```python
from build123d import *

# Parameters (mm, degrees)
EXTRUDE_1_DEPTH             = 90
SKETCH_2_W                  = 90
SKETCH_2_H                  = 17.75
EXTRUDE_2_DEPTH             = 8.2
SKETCH_3_W                  = 90
SKETCH_3_H                  = 50.95
EXTRUDE_3_DEPTH             = 8.2
SKETCH_4_W                  = 3.95
SKETCH_4_H                  = 29.5
CUT_EXTRUDE_1_DEPTH         = 91
SKETCH_5_W                  = 3.95
SKETCH_5_H                  = 6.2
CUT_EXTRUDE_2_DEPTH         = 91
SKETCH_6_W                  = 2.25
SKETCH_6_H                  = 3.95
CUT_EXTRUDE_3_DEPTH         = 91
SKETCH_7_W                  = 4.5
SKETCH_7_H                  = 3.95
CUT_EXTRUDE_4_DEPTH         = 91
SKETCH_8_W                  = 2.25
SKETCH_8_H                  = 3.95
CUT_EXTRUDE_5_DEPTH         = 91
SKETCH_9_W                  = 3.95
SKETCH_9_H                  = 2.25
CUT_EXTRUDE_6_DEPTH         = 91
SKETCH_10_W                 = 19.6
SKETCH_10_H                 = 44.6
CUT_EXTRUDE_7_DEPTH         = 86.2
HOLE_WIZARD_2_5_2_5_1_D     = 2.5
HOLE_WIZARD_2_5_2_5_1_DEPTH = 90
HOLE_WIZARD_4_5_4_5_1_D     = 4.5
HOLE_WIZARD_4_5_4_5_1_DEPTH = 90
FILLET_1_R                  = 2
FILLET_2_R                  = 2
SKETCH_17_R                 = 1.25
EXTRUDE_4_DEPTH             = 90


with BuildPart() as part:
    # Эскиз1 → Бобышка-Вытянуть1 (new body)
    with BuildSketch(Plane(origin=(90, 0, 0), x_dir=(0, 0, -1), z_dir=(1, 0, 0))):
        with BuildLine():
            Line((6.75, -24.093761792), (6.75, 19.25))
            Line((6.75, 19.25), (-11.593761792, 19.25))
            ThreePointArc((-11.593761792, 19.25), (-15.325, 18), (-11.593761792, 16.75))
            Line((-11.593761792, 16.75), (-11, 16.75))
            Line((-11, 16.75), (-11, -16.75))
            Line((-11, -16.75), (-11.593761792, -16.75))
            ThreePointArc((-11.593761792, -16.75), (-15.325, -18), (-11.593761792, -19.25))
            Line((-11.593761792, -19.25), (-11, -19.25))
            Line((-11, -19.25), (-11, -23.5))
            Line((-11, -23.5), (-6.75, -23.5))
            Line((-6.75, -23.5), (-6.75, -24.093761792))
            ThreePointArc((-6.75, -24.093761792), (-5.5, -27.825), (-4.25, -24.093761792))
            Line((-4.25, -24.093761792), (-4.25, -23.5))
            Line((-4.25, -23.5), (4.25, -23.5))
            Line((4.25, -23.5), (4.25, -24.093761792))
            ThreePointArc((4.25, -24.093761792), (5.5, -27.825), (6.75, -24.093761792))
        make_face()
    extrude(amount=-EXTRUDE_1_DEPTH)

    # Эскиз2 → Бобышка-Вытянуть2 (add)
    with BuildSketch(Plane(origin=(0, 19.25, 0), x_dir=(-1, 0, 0), z_dir=(0, 1, 0))):
        with Locations((-45, 2.125)):
            Rectangle(SKETCH_2_W, SKETCH_2_H)
    extrude(amount=EXTRUDE_2_DEPTH)

    # Эскиз3 → Бобышка-Вытянуть3 (add)
    with BuildSketch(Plane(origin=(0, 0, -6.75), x_dir=(-1, 0, 0), z_dir=(0, 0, -1))):
        with Locations((-45, 1.975)):
            Rectangle(SKETCH_3_W, SKETCH_3_H)
    extrude(amount=EXTRUDE_3_DEPTH)

    # Эскиз4 → Вырез-Вытянуть1 (cut, through all)
    with BuildSketch(Plane.ZY):
        with Locations((-12.975, 0)):
            Rectangle(SKETCH_4_W, SKETCH_4_H)
    extrude(amount=-CUT_EXTRUDE_1_DEPTH, mode=Mode.SUBTRACT)

    # Эскиз5 → Вырез-Вытянуть2 (cut, through all)
    with BuildSketch(Plane.ZY):
        with Locations((-12.975, 24.35)):
            Rectangle(SKETCH_5_W, SKETCH_5_H)
    extrude(amount=-CUT_EXTRUDE_2_DEPTH, mode=Mode.SUBTRACT)

    # Эскиз6 → Вырез-Вытянуть3 (cut, through all)
    with BuildSketch(Plane.ZY):
        with Locations((-9.875, 25.475)):
            Rectangle(SKETCH_6_W, SKETCH_6_H)
    extrude(amount=-CUT_EXTRUDE_3_DEPTH, mode=Mode.SUBTRACT)

    # Эскиз7 → Вырез-Вытянуть4 (cut, through all)
    with BuildSketch(Plane.ZY):
        with Locations((0, 25.475)):
            Rectangle(SKETCH_7_W, SKETCH_7_H)
    extrude(amount=-CUT_EXTRUDE_4_DEPTH, mode=Mode.SUBTRACT)

    # Эскиз8 → Вырез-Вытянуть5 (cut, through all)
    with BuildSketch(Plane.ZY):
        with Locations((9.875, 25.475)):
            Rectangle(SKETCH_8_W, SKETCH_8_H)
    extrude(amount=-CUT_EXTRUDE_5_DEPTH, mode=Mode.SUBTRACT)

    # Эскиз9 → Вырез-Вытянуть6 (cut, through all)
    with BuildSketch(Plane.ZY):
        with Locations((-12.975, -22.375)):
            Rectangle(SKETCH_9_W, SKETCH_9_H)
    extrude(amount=-CUT_EXTRUDE_6_DEPTH, mode=Mode.SUBTRACT)

    # Эскиз10 → Вырез-Вытянуть7 (cut)
    with BuildSketch(Plane(origin=(90, 0, 0), x_dir=(0, 0, -1), z_dir=(1, 0, 0))):
        Rectangle(SKETCH_10_W, SKETCH_10_H)
    extrude(amount=-CUT_EXTRUDE_7_DEPTH, mode=Mode.SUBTRACT)

    # Диаметр отверстия Ø2.5 (2.5)1
    with Locations(Plane(origin=(90, 0, 0), x_dir=(0, 0, -1), z_dir=(1, 0, 0))):
        with Locations((5.5, -25.75), (-13.25, -18), (-5.5, -25.75), (-13.25, 18)):
            Hole(HOLE_WIZARD_2_5_2_5_1_D / 2, depth=HOLE_WIZARD_2_5_2_5_1_DEPTH)

    # Диаметр отверстия Ø4.5 (4.5)1
    with Locations(Plane.ZY):
        with Locations((-13.25, -18), (-13.25, 18), (-5.5, 25.75), (5.5, 25.75)):
            Hole(HOLE_WIZARD_4_5_4_5_1_D / 2, depth=HOLE_WIZARD_4_5_4_5_1_DEPTH)

    # Скругление1
    fillet_1_edges = [part.edges().sort_by_distance(p)[0] for p in [
        (45, 23.5, 8.75),
    ]]
    fillet(fillet_1_edges, radius=FILLET_1_R)

    # Скругление2
    fillet_2_edges = [part.edges().sort_by_distance(p)[0] for p in [
        (45, 23.5, -8.75),
        (45, 23.5, 2.25),
        (45, 23.5, -2.25),
        (45, -21.25, -11),
        (45, 14.75, -11),
        (45, -14.75, -11),
        (45, 21.25, -11),
    ]]
    fillet(fillet_2_edges, radius=FILLET_2_R)

    # Эскиз17 → Бобышка-Вытянуть4 (add)
    with BuildSketch(Plane(origin=(90, 0, 0), x_dir=(0, 0, -1), z_dir=(1, 0, 0))):
        with Locations((5.5, -25.75)):
            Circle(SKETCH_17_R)
        with Locations((-5.5, -25.75)):
            Circle(SKETCH_17_R)
        with Locations((-13.25, -18)):
            Circle(SKETCH_17_R)
        with Locations((-13.25, 18)):
            Circle(SKETCH_17_R)
    extrude(amount=-EXTRUDE_4_DEPTH)


solid = part.part
```
Part model, mm, in its own coordinate system. A direction names the side the tool comes from. Round coordinates to 2 decimals unless told otherwise and drop trailing zeros. Order: outer loops, then holes, each group sorted by start corner. A loop starts at its lowest first (then second) coordinate and runs counter-clockwise, first axis right, second up. Notation, with made-up numbers: M 88.5,56 L 130.5,56 A12 cw 130.5,64 Z; hole C 0.25,52.5 d11. An arc over 180 degrees is marked long. Answer in a Markdown table with one row per item. Add a question column.
Q1. Cut at C-C on y = -6. Give the cut face in (x, z).
Q2. Cut at B-B on z = 13.25. Give the cut face in (x, y) (3 decimals).
Q3. 3-axis set-ups, long thin cutter, end or side, ignore diameter. For faces 1 (the face through (46, 21, 11)), 2 (the face through (45.63, -14.15, -11.57)), 3 (the face through (46, -23.5, 0)): which of +Z, -Z, +X, -X, +Y, -Y reach the whole face in a straight line?
Q4. Mould opens along Z. For faces 4 (the face through (48, 22.3, 0)), 5 (the face through (44, 26, -8.75)), 6 (the face through (44, 26, 8.75)), 7 (the face through (0, -1, 0)) say: +Z half, -Z half, draft (parallel to the pull), parting line (faces both ways), or undercut.
Q5. Cut at A-A on y = -25.75. Give the cut face in (x, z) (3 decimals), and give its area (3 significant figures).
Q6. Wall check: L1, parallel to Y at x = 44, z = -13.25; L2, parallel to Z at x = 29, y = 25.75; L3, parallel to Y at x = 50, z = -13. Give the ranges that are in metal, low to high. Write a range as from..to.
Q7. Cut at D-D on z = -5.5. Give the cut face in (x, y) (3 decimals).
Q8. Pin check, flat tips, straight feed: pin 1 (1.6 mm diameter, centred on x = 64.5, z = -14, fed in from +Y); pin 2 (6 mm diameter, centred on y = 14, z = -3.5, fed in from -X); pin 3 (2 mm diameter, centred on x = 16.5, z = -2, fed in from -Y); pin 4 (13 mm diameter, centred on x = 43.5, y = -2, fed in from -Z). Stop position of each tip, or through.
Established:
| question | item | result |
|---|---|---|
| 1 | outline | M 0,-11 L 90,-11 L 90,-9.8 L 3.8,-9.8 L 3.8,9.8 L 90,9.8 L 90,11 L 0,11 Z |
| 2 | outline | M 0,-20.075 L 90,-20.075 L 90,-15.925 L 0,-15.925 Z; M 0,15.925 L 90,15.925 L 90,20.075 L 0,20.075 Z |
| 3 | face 1 | +X, -X, +Y |
| 3 | face 2 | -Z, +X, -X |
| 3 | face 3 | +X, -X |
| 4 | face 4 | undercut |
| 4 | face 5 | -Z half |
| 4 | face 6 | +Z half |
| 4 | face 7 | draft |
| 5 | outline | M 0,-7.575 L 90,-7.575 L 90,-3.425 L 0,-3.425 Z; M 0,3.425 L 90,3.425 L 90,7.575 L 0,7.575 Z |
| 5 | area | 747 mm2 |
| 6 | L1 | y = -21.25..-20.25, -15.75..-14.75, 14.75..15.75, 20.25..21.25 |
| 6 | L2 | z = -8.75..-7.75, -3.25..-2.25, 2.25..3.25, 7.75..8.75 |
| 6 | L3 | y = -21.25..-20.24, -15.76..-14.75, 14.75..15.76, 20.24..21.25 |
| 7 | outline | M 0,-27.825 L 90,-27.825 L 90,-22.3 L 3.8,-22.3 L 3.8,22.3 L 90,22.3 L 90,23.5 L 0,23.5 Z |
| 8 | pin 1 | stops at y = 21.25 |
| 8 | pin 2 | stops at x = 0 |
| 8 | pin 3 | stops at y = -23.5 |
| 8 | pin 4 | stops at z = -11 |
